Could you check a few things on this model? Use its own coordinates, in mm. Face numbers are marked on the shaded views. Round coordinates to 2 decimals unless told otherwise and drop trailing zeros. Loops run counter-clockwise (first coordinate to the right, second up) from the corner with the lowest first, then second, coordinate; pieces in that order, holes last. Notation, with made-up numbers: (88.25, 23.5) -> (142.25, 23.5) arc R26 cw to (142.25, 50.5) -> close; hole circle Ø10 at (56, 56.25). An arc over 180 degrees is marked (long way). One line per item, written item: value.
```python
from build123d import *

# Parameters (mm, degrees)
ESQUISSE1_R                  = 17
ESQUISSE1_R_2                = 10
EXTRUSION1_DEPTH             = 5
ESQUISSE2_R                  = 2.1
ENL_V_MAT_EXTRU_1_DEPTH      = 25.556058316
R_P_TITION_CIRCULAIRE1_COUNT = 4


with BuildPart() as part:
    # Esquisse1 → Extrusion1 (new body)
    with BuildSketch(Plane.XY):
        Circle(ESQUISSE1_R)
        Circle(ESQUISSE1_R_2, mode=Mode.SUBTRACT)
    extrude(amount=EXTRUSION1_DEPTH)

    # Esquisse2 → Enl_v. mat.-Extru.1 (cut, through all)
    with BuildSketch(Plane.XY.offset(5)):
        with Locations((0, 13)):
            Circle(ESQUISSE2_R)
    enl_v_mat_extru_1 = extrude(amount=-ENL_V_MAT_EXTRU_1_DEPTH, mode=Mode.SUBTRACT)

    # R_p_tition circulaire1: Enl_v. mat.-Extru.1 ×4 about axis
    r_p_tition_circulaire1_axis = Axis((0, 0, 0), (0, 0, 1))
    for i in range(1, R_P_TITION_CIRCULAIRE1_COUNT):
        add(enl_v_mat_extru_1.rotate(r_p_tition_circulaire1_axis, i * 360 / R_P_TITION_CIRCULAIRE1_COUNT), mode=Mode.SUBTRACT)


solid = part.part
```
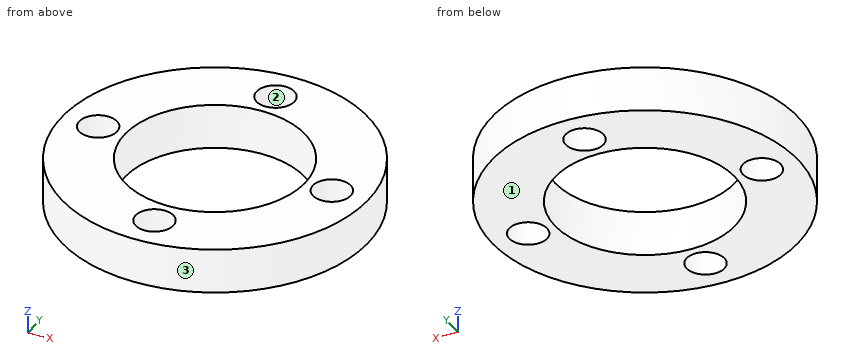
(1) Please list where these lines run through material, in increasing order: L1, parallel to Y at x = 0, z = 1.25; L2, parallel to X at y = 1.5, z = 1.85; L3, parallel to Y at x = 1, z = 0.8.
Results below:
L1: y = -17 to -15.1, -10.9 to -10, 10 to 10.9, 15.1 to 17
L2: x = -16.93 to -14.47, -11.53 to -9.89, 9.89 to 11.53, 14.47 to 16.93
L3: y = -16.97 to -14.85, -11.15 to -9.95, 9.95 to 11.15, 14.85 to 16.97
(2) Imagine slicing it at A-A on x = 0. Write out the boundary of the cut face in (y, z), then the cut area to 3 significant figures.
Results below:
outline: (-17, 0) -> (-15.1, 0) -> (-15.1, 5) -> (-17, 5) -> close; (-10.9, 0) -> (-10, 0) -> (-10, 5) -> (-10.9, 5) -> close; (10, 0) -> (10.9, 0) -> (10.9, 5) -> (10, 5) -> close; (15.1, 0) -> (17, 0) -> (17, 5) -> (15.1, 5) -> close
area: 28.0 mm²
(3) For pin 1 Ø3 at (x, y) = (10, -1.5) entering from -Z; pin 2 Ø1 at (x, z) = (5, 4) entering from -Y; pin 3 Ø3 at (y, z) = (12, 1) entering from -X, each with a flat end and sliding along its axis, tell me the tip position at first contact or that it passes through.
Results below:
pin 1: stops at z = 0
pin 2: stops at y = -16.39
pin 3: stops at x = -13.37
(4) Imagine slicing it at D-D on z = 1.5. Write out the boundary of the cut face in (x, y).
Results below:
outline: circle Ø34 at (0, 0); hole circle Ø4.2 at (-13, 0); hole circle Ø20 at (0, 0); hole circle Ø4.2 at (0, -13); hole circle Ø4.2 at (0, 13); hole circle Ø4.2 at (13, 0)
(5) Imagine slicing it at C-C on x = -14. Write out the boundary of the cut face in (y, z), then the cut area to 3 significant figures.
Results below:
outline: (-9.64, 0) -> (-1.85, 0) -> (-1.85, 5) -> (-9.64, 5) -> close; (1.85, 0) -> (9.64, 0) -> (9.64, 5) -> (1.85, 5) -> close
area: 78.0 mm²
(6) We'd pull the mould along Y, two halves only. Please class the marked faces 1, 2 and 3: +Y half, -Y half, draft (parallel to the pull), parting line (faces both ways), or undercut.
Results below:
face 1: draft
face 2: undercut
face 3: parting line
